Build history of the part. All positions in model axes, mm. Face numbers are marked on the shaded views. A direction names the side the tool comes from. Coordinates: 2 decimals unless noted, no trailing zeros. Loops run counter-clockwise (first coordinate to the right, second up) from the corner with the lowest first, then second, coordinate; pieces in that order, holes last.
(1) Slice it at B-B (z = 6). Give the cut face in (x, y).
(2) Flat gauge pins, fed straight in: P1, Ø1.5, axis at x = -2.5, z = 8, coming from the +Y side; P2, Ø5, axis at y = 2.98, z = 0, coming from the +X side; P3, Ø3, axis at x = -3, y = 33, coming from the -Z side; P4, Ø1.5, axis at x = -0.5, y = 24.5, coming from the -Z side. Where does each tip first touch, or does it go through?
(3) Wall check: L1, parallel to Z at x = -1.95, y = 11.5; L2, parallel to Y at x = -2.7, z = 7.25; L3, parallel to Y at x = -0.95, z = 3.5. Give the ranges that are in metal, low to high.
(4) Tool access for the marked faces 4, 5 and 6: list every direction of +Z, -Z, +X, -X, +Y, -Y with a clear straight run to the whole face (end or side of a thin tool).
(5) Slice it at A-A (y = 2). Give the cut face in (x, z), and give its area (3 significant figures).
(6) Slice it at C-C (y = 16). Give the cut face in (x, z), and give its area (3 significant figures).
(7) Two-plate mould, pull along Z, no slides. Class the marked faces 1, 2 and 3: pulls with the +Z half, pulls with the -Z half, needs draft (parallel to the pull), parting line crosses it, or undercut.
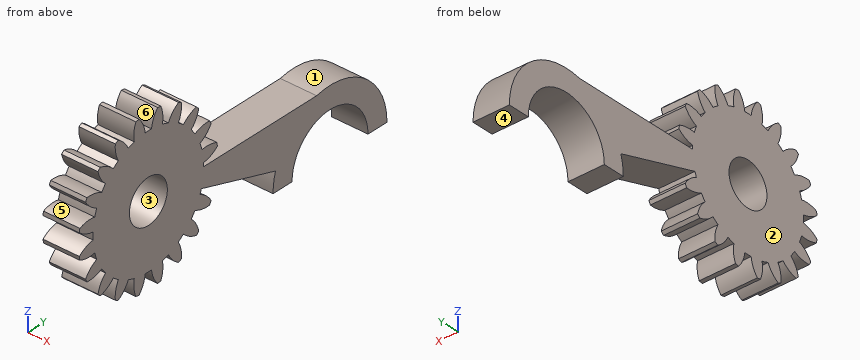
from build123d import *

# Parameters (mm, degrees)
SKETCH_2_R      = 3
EXTRUDE_2_DEPTH = 5


with BuildPart() as part:
    # ｽｹｯﾁ2 → ﾎﾞｽ - 押し出し2 (new body)
    with BuildSketch(Plane(origin=(-4.158413815, 0, 0), x_dir=(0, 0, -1), z_dir=(1, 0, 0))):
        with BuildLine():
            Line((8.749, 22.67838595), (8.749, 25.67838595))
            ThreePointArc((8.749, 25.67838595), (2.749, 31.67838595), (8.749, 37.67838595))
            Line((8.749, 37.67838595), (8.749, 40.67838595))
            ThreePointArc((8.749, 40.67838595), (1.678067187, 37.246321757), (0, 29.567699095))
            Line((0, 29.567699095), (0, 11.731480336))
            ThreePointArc((0, 11.731480336), (-0.250064167, 11.727905936), (-0.499924007, 11.717185654))
            ThreePointArc((-0.499924007, 11.717185654), (-0.818060825, 12.87403268), (-1.464956435, 13.884494033))
            ThreePointArc((-1.464956435, 13.884494033), (-1.720779115, 13.847052083), (-1.975651141, 13.803607938))
            ThreePointArc((-1.975651141, 13.803607938), (-2.278635697, 12.642700346), (-2.223716399, 11.444163761))
            ThreePointArc((-2.223716399, 11.444163761), (-2.703589684, 11.303273797), (-3.174628369, 11.135193732))
            ThreePointArc((-3.174628369, 11.135193732), (-3.834679853, 12.137110952), (-4.762163869, 12.898215069))
            ThreePointArc((-4.762163869, 12.898215069), (-4.993895497, 12.783552102), (-5.222868219, 12.663474478))
            ThreePointArc((-5.222868219, 12.663474478), (-5.15228348, 11.465758371), (-4.729683951, 10.342853338))
            ThreePointArc((-4.729683951, 10.342853338), (-5.142533172, 10.06057002), (-5.538577987, 9.75515742))
            ThreePointArc((-5.538577987, 9.75515742), (-6.4759337, 10.504070195), (-7.593217523, 10.941314902))
            ThreePointArc((-7.593217523, 10.941314902), (-7.778174593, 10.760654929), (-7.958834566, 10.57569786))
            ThreePointArc((-7.958834566, 10.57569786), (-7.521589858, 9.458414036), (-6.772677084, 8.521058323))
            ThreePointArc((-6.772677084, 8.521058323), (-7.078089684, 8.125013509), (-7.360373002, 7.712164287))
            ThreePointArc((-7.360373002, 7.712164287), (-8.483278035, 8.134763816), (-9.680994141, 8.205348555))
            ThreePointArc((-9.680994141, 8.205348555), (-9.801071766, 7.976375833), (-9.915734733, 7.744644205))
            ThreePointArc((-9.915734733, 7.744644205), (-9.154630615, 6.81716019), (-8.152713396, 6.157108705))
            ThreePointArc((-8.152713396, 6.157108705), (-8.320793461, 5.68607002), (-8.461683425, 5.206196735))
            ThreePointArc((-8.461683425, 5.206196735), (-9.66022001, 5.261116033), (-10.821127601, 4.958131478))
            ThreePointArc((-10.821127601, 4.958131478), (-10.864571747, 4.703259452), (-10.902013697, 4.447436771))
            ThreePointArc((-10.902013697, 4.447436771), (-9.891552344, 3.800541161), (-8.734705318, 3.482404344))
            ThreePointArc((-8.734705318, 3.482404344), (-8.749, 2.982480336), (-8.734705318, 2.482556329))
            ThreePointArc((-8.734705318, 2.482556329), (-9.891552344, 2.164419511), (-10.902013697, 1.517523901))
            ThreePointArc((-10.902013697, 1.517523901), (-10.864571747, 1.261701221), (-10.821127601, 1.006829195))
            ThreePointArc((-10.821127601, 1.006829195), (-9.66022001, 0.70384464), (-8.461683425, 0.758763937))
            ThreePointArc((-8.461683425, 0.758763937), (-8.320793461, 0.278890652), (-8.152713396, -0.192148033))
            ThreePointArc((-8.152713396, -0.192148033), (-9.154630615, -0.852199517), (-9.915734733, -1.779683533))
            ThreePointArc((-9.915734733, -1.779683533), (-9.801071766, -2.011415161), (-9.680994141, -2.240387883))
            ThreePointArc((-9.680994141, -2.240387883), (-8.483278035, -2.169803144), (-7.360373002, -1.747203615))
            ThreePointArc((-7.360373002, -1.747203615), (-7.078089684, -2.160052836), (-6.772677084, -2.556097651))
            ThreePointArc((-6.772677084, -2.556097651), (-7.521589858, -3.493453364), (-7.958834566, -4.610737187))
            ThreePointArc((-7.958834566, -4.610737187), (-7.778174593, -4.795694257), (-7.593217523, -4.976354229))
            ThreePointArc((-7.593217523, -4.976354229), (-6.4759337, -4.539109522), (-5.538577987, -3.790196748))
            ThreePointArc((-5.538577987, -3.790196748), (-5.142533172, -4.095609348), (-4.729683951, -4.377892665))
            ThreePointArc((-4.729683951, -4.377892665), (-5.15228348, -5.500797699), (-5.222868219, -6.698513805))
            ThreePointArc((-5.222868219, -6.698513805), (-4.993895497, -6.81859143), (-4.762163869, -6.933254396))
            ThreePointArc((-4.762163869, -6.933254396), (-3.834679853, -6.172150279), (-3.174628369, -5.17023306))
            ThreePointArc((-3.174628369, -5.17023306), (-2.703589684, -5.338313125), (-2.223716399, -5.479203088))
            ThreePointArc((-2.223716399, -5.479203088), (-2.278635697, -6.677739674), (-1.975651141, -7.838647265))
            ThreePointArc((-1.975651141, -7.838647265), (-1.720779115, -7.88209141), (-1.464956435, -7.91953336))
            ThreePointArc((-1.464956435, -7.91953336), (-0.818060825, -6.909072007), (-0.499924007, -5.752224981))
            ThreePointArc((-0.499924007, -5.752224981), (0, -5.766519664), (0.499924007, -5.752224981))
            ThreePointArc((0.499924007, -5.752224981), (0.818060825, -6.909072007), (1.464956435, -7.91953336))
            ThreePointArc((1.464956435, -7.91953336), (1.720779115, -7.88209141), (1.975651141, -7.838647265))
            ThreePointArc((1.975651141, -7.838647265), (2.278635697, -6.677739674), (2.223716399, -5.479203088))
            ThreePointArc((2.223716399, -5.479203088), (2.703589684, -5.338313125), (3.174628369, -5.17023306))
            ThreePointArc((3.174628369, -5.17023306), (3.834679853, -6.172150279), (4.762163869, -6.933254396))
            ThreePointArc((4.762163869, -6.933254396), (4.993895497, -6.81859143), (5.222868219, -6.698513805))
            ThreePointArc((5.222868219, -6.698513805), (5.15228348, -5.500797699), (4.729683951, -4.377892665))
            ThreePointArc((4.729683951, -4.377892665), (5.142533172, -4.095609348), (5.538577987, -3.790196748))
            ThreePointArc((5.538577987, -3.790196748), (6.4759337, -4.539109522), (7.593217523, -4.976354229))
            ThreePointArc((7.593217523, -4.976354229), (7.778174593, -4.795694257), (7.958834566, -4.610737187))
            ThreePointArc((7.958834566, -4.610737187), (7.521589858, -3.493453364), (6.772677084, -2.556097651))
            ThreePointArc((6.772677084, -2.556097651), (7.078089684, -2.160052836), (7.360373002, -1.747203615))
            ThreePointArc((7.360373002, -1.747203615), (8.483278035, -2.169803144), (9.680994141, -2.240387883))
            ThreePointArc((9.680994141, -2.240387883), (9.801071766, -2.011415161), (9.915734733, -1.779683533))
            ThreePointArc((9.915734733, -1.779683533), (9.154630615, -0.852199517), (8.152713396, -0.192148033))
            ThreePointArc((8.152713396, -0.192148033), (8.320793461, 0.278890652), (8.461683425, 0.758763937))
            ThreePointArc((8.461683425, 0.758763937), (9.66022001, 0.70384464), (10.821127601, 1.006829195))
            ThreePointArc((10.821127601, 1.006829195), (10.864571747, 1.261701221), (10.902013697, 1.517523901))
            ThreePointArc((10.902013697, 1.517523901), (9.891552344, 2.164419511), (8.734705318, 2.482556329))
            ThreePointArc((8.734705318, 2.482556329), (8.749, 2.982480336), (8.734705318, 3.482404344))
            ThreePointArc((8.734705318, 3.482404344), (9.891552344, 3.800541161), (10.902013697, 4.447436771))
            ThreePointArc((10.902013697, 4.447436771), (10.864571747, 4.703259452), (10.821127601, 4.958131478))
            ThreePointArc((10.821127601, 4.958131478), (9.66022001, 5.261116033), (8.461683425, 5.206196735))
            ThreePointArc((8.461683425, 5.206196735), (8.320793461, 5.68607002), (8.152713396, 6.157108705))
            ThreePointArc((8.152713396, 6.157108705), (9.154630615, 6.81716019), (9.915734733, 7.744644205))
            ThreePointArc((9.915734733, 7.744644205), (9.801071766, 7.976375833), (9.680994141, 8.205348555))
            ThreePointArc((9.680994141, 8.205348555), (8.483278035, 8.134763816), (7.360373002, 7.712164287))
            ThreePointArc((7.360373002, 7.712164287), (7.078089684, 8.125013509), (6.772677084, 8.521058323))
            ThreePointArc((6.772677084, 8.521058323), (7.521589858, 9.458414036), (7.958834566, 10.57569786))
            ThreePointArc((7.958834566, 10.57569786), (7.778174593, 10.760654929), (7.593217523, 10.941314902))
            ThreePointArc((7.593217523, 10.941314902), (6.4759337, 10.504070195), (5.538577987, 9.75515742))
            ThreePointArc((5.538577987, 9.75515742), (5.142533172, 10.06057002), (4.729683951, 10.342853338))
            ThreePointArc((4.729683951, 10.342853338), (5.15228348, 11.465758371), (5.222868219, 12.663474478))
            ThreePointArc((5.222868219, 12.663474478), (4.993895497, 12.783552102), (4.762163869, 12.898215069))
            ThreePointArc((4.762163869, 12.898215069), (3.834679853, 12.137110952), (3.174628369, 11.135193732))
            ThreePointArc((3.174628369, 11.135193732), (2.865099875, 11.249051796), (2.551500033, 11.351162943))
            Line((2.551500033, 11.351162943), (6.1243, 23.069614266))
            ThreePointArc((6.1243, 23.069614266), (7.422151319, 22.776730341), (8.749, 22.67838595))
        make_face()
        with Locations(Location((0, 2.982480336, 0), (0, 0, 180))):
            Circle(SKETCH_2_R, mode=Mode.SUBTRACT)
    extrude(amount=EXTRUDE_2_DEPTH)


solid = part.part
Response values:
1. outline: (-4.16, -4.22) - (0.84, -4.22) - (0.84, 10.18) - (-4.16, 10.18) - close
2. P1: stops at y = 10.94
2. P2: passes through
2. P3: stops at z = -3.45
2. P4: stops at z = -8.75
3. L1: z = -5.16 to -3.37, -2.6 to 2.23, 3.37 to 5.16
3. L2: y = -4.88 to -3.08, -1.91 to 7.88, 9.05 to 10.85
3. L3: y = -5.75 to 11.71
4. face 4: -Z, +X, -X, +Y
4. face 5: +X, -X
4. face 6: +Z, +X, -X
5. outline: (-4.16, -10.22) - (0.84, -10.22) - (0.84, -2.83) - (-4.16, -2.83) - close; (-4.16, 2.83) - (0.84, 2.83) - (0.84, 10.22) - (-4.16, 10.22) - close
5. area: 73.8 mm2
6. outline: (-4.16, -3.97) - (0.84, -3.97) - (0.84, 0) - (-4.16, 0) - close
6. area: 19.8 mm2
7. face 1: pulls with the +Z half
7. face 2: needs draft
7. face 3: undercut
